Work out the finished part from the listing and answer in its coordinate system (mm). A direction names the side the tool comes from. Coordinates: 2 decimals unless noted, no trailing zeros. Use a Markdown table: item, result. Add a question column.
(1) Given pin 1 Ø1.5 at (y, z) = (145.5, 31) entering from -X, flat-ended and moving along its own axis, determine where the tip first touches the part or whether it passes through.
(2) For a pull along X with two mould halves and no side action, classify faces 3 (the face through (0, 182, 14)), 4 (the face through (156.27, 59.63, 11.81)), 5 (the face through (338, 187, 0)), 6 (the face through (163.071, 345.707, 23.746)) as released by +X, released by -X, zero draft, split by the parting line, or undercut.
(3) A tool of negligible diameter and unlimited length cuts with its end or side. For faces 1 (the face through (275, 368.3, 19)), 2 (the face through (231, 306, 19.05)), from which of +Z, -Z, +X, -X, +Y, -Y can it reach the whole face along a straight path? Write none if from no direction.
(4) Find the intervals of material crossed by line 1 (Y direction, x = 184, z = 21); line 2 (Y direction, x = 184.15, z = 13.5); line 3 (X direction, y = 150.5, z = 31), in increasing order. Write a range as from..to.
from build123d import *

# Parameters (mm, degrees)
F0_W     = 558.8
F0_H     = 368.3
F0_R     = 161.925
F1_DEPTH = 38.1
F0_R_2   = 128.5875
F2_DEPTH = 19.05
F3_R     = 9.525
F4_R     = 4.7625
F5_R     = 9.525


with BuildPart() as f1:
    # F0 (on Top) → F1 (new body)
    with BuildSketch(Plane.XY):
        with Locations((279.4, 184.15)):
            Rectangle(F0_W, F0_H)
        with Locations((184.15, 185.159966)):
            Circle(F0_R, mode=Mode.SUBTRACT)
    extrude(amount=F1_DEPTH)

    # F0 (on Top) → F2 (join)
    with BuildSketch(Plane.XY):
        with Locations((184.15, 185.159966)):
            Circle(F0_R)
        with Locations((184.15, 185.159966)):
            Circle(F0_R_2, mode=Mode.SUBTRACT)
    extrude(amount=F2_DEPTH)

    # F3
    f3_edges = [f1.edges().sort_by_distance(p)[0] for p in [
        (22.225, 185.159966, 38.1),
    ]]
    fillet(f3_edges, radius=F3_R)

    # F4
    f4_edges = [f1.edges().sort_by_distance(p)[0] for p in [
        (55.5625, 185.159966, 0),
    ]]
    fillet(f4_edges, radius=F4_R)

    # F5
    f5_edges = [f1.edges().sort_by_distance(p)[0] for p in [
        (558.8, 184.15, 38.1),
        (0, 184.15, 38.1),
    ]]
    fillet(f5_edges, radius=F5_R)


solid = f1.part
Model answer:
| question | item | result |
|---|---|---|
| 1 | pin 1 | x = 0.15 |
| 2 | face 3 | released by -X |
| 2 | face 4 | undercut |
| 2 | face 5 | zero draft |
| 2 | face 6 | undercut |
| 3 | face 1 | +Z, -Z, +X, -X, +Y |
| 3 | face 2 | +Z |
| 4 | line 1 | 0..23.24, 347.08..368.3 |
| 4 | line 2 | 0..56.57, 313.75..368.3 |
| 4 | line 3 | 0.31..25.66, 342.64..558.49 |
